Build history of the part. All positions in model axes, mm. A direction names the side the tool comes from. Give positions to 0.01 mm unless a question says otherwise; leave off trailing zeros. Write item = value, one per line. Start each with the question number.
Q1. Mould opens along Y. For faces 1 (the face through (62.12, 0.04, 3.13)), 2 (the face through (-12.17, 78.12, 3.13)), 3 (the face through (-38.56, 46.17, 3.13)), 4 (the face through (1, 3, 6.35)) say: pulls with the +Y half, pulls with the -Y half, needs draft (parallel to the pull), parting line crosses it, or undercut.
Q2. Drop flat-ended pins along their axis: P1, Ø4, axis at x = -28.5, y = -54.2, coming from the -Z side; P2, Ø2, axis at x = -41.5, z = 5.5, coming from the +Y side; P3, Ø3, axis at x = 43.5, z = 4.5, coming from the +Y side. Give the stop position or say it passes through.
Q3. Tool access for faces 5 (the face through (1, 3, 0)), 6 (the face through (-33.757, -32.465, 3.131)): list every direction of +Z, -Z, +X, -X, +Y, -Y with a clear straight run to the whole face (end or side of a thin tool).
Q4. Wall check: line 1 (X direction, y = -31, z = 3.5); line 2 (Y direction, x = -18.5, z = 4.5); line 3 (Y direction, x = 28, z = 5). Give the ranges that are in metal, low to high.
Q5. Saw through at A-A, the plane z = 1.25. Give the number of separate pieces and of enclosed holes in the cut face, then the cut area to 3 significant figures.
from build123d import *

# Parameters (mm, degrees)
MODEL_R             = 1.45
MODEL_R_2           = 1.55
MODEL_R_3           = 3.3
MODEL_R_4           = 3.048
BOSS_EXTRUDE1_DEPTH = 6.35


with BuildPart() as part:
    # Model → Boss-Extrude1 (new body)
    with BuildSketch(Plane.XY):
        with BuildLine():
            ThreePointArc((71.963132539, -16.30426092), (71.896606956, -19.345127891), (73.024752162, -22.169766979))
            ThreePointArc((73.024752162, -22.169766979), (73.705673151, -28.611226497), (68.857053859, -32.906217194))
            ThreePointArc((68.857053859, -32.906217194), (66.118599711, -34.22991144), (64.11603721, -36.519243442))
            ThreePointArc((64.11603721, -36.519243442), (11.268864031, -72.921423961), (-50.101470416, -54.169770455))
            ThreePointArc((-50.101470416, -54.169770455), (-52.70167567, -52.591724124), (-55.71195748, -52.156406987))
            ThreePointArc((-55.71195748, -52.156406987), (-61.630885553, -49.525372103), (-62.92614696, -43.178849276))
            ThreePointArc((-62.92614696, -43.178849276), (-62.703272731, -40.145431292), (-63.684611152, -37.266495293))
            ThreePointArc((-63.684611152, -37.266495293), (-68.786237646, 26.701589457), (-21.861662123, 70.474031375))
            ThreePointArc((-21.861662123, 70.474031375), (-19.194931286, 71.936852015), (-17.312794682, 74.326173966))
            ThreePointArc((-17.312794682, 74.326173966), (-12.074787597, 78.1365986), (-5.930906899, 76.08506647))
            ThreePointArc((-5.930906899, 76.08506647), (-3.41532698, 74.375342732), (-0.431426057, 73.785738734))
            ThreePointArc((-0.431426057, 73.785738734), (57.517373614, 46.219834503), (71.963132539, -16.30426092))
        make_face()
        with Locations((-10.994529329, 71.146189371)):
            Circle(MODEL_R, mode=Mode.SUBTRACT)
        with Locations((-56.117142713, -45.094636387)):
            Circle(MODEL_R, mode=Mode.SUBTRACT)
        with Locations((-4.695418168, 60.932414429)):
            Circle(MODEL_R, mode=Mode.SUBTRACT)
        with Locations((-31.422079216, 58.547967052)):
            Circle(MODEL_R, mode=Mode.SUBTRACT)
        with Locations((-25.122968055, 48.33419211)):
            Circle(MODEL_R, mode=Mode.SUBTRACT)
        with Locations((-50.421309724, -34.532558628)):
            Circle(MODEL_R, mode=Mode.SUBTRACT)
        with Locations((-34.9929872, -56.486302366)):
            Circle(MODEL_R, mode=Mode.SUBTRACT)
        with Locations((-29.29715421, -45.924224608)):
            Circle(MODEL_R, mode=Mode.SUBTRACT)
        with Locations((67.111672043, -26.051552984)):
            Circle(MODEL_R, mode=Mode.SUBTRACT)
        with Locations((-24.235417087, 18.341485339)):
            Circle(MODEL_R_2, mode=Mode.SUBTRACT)
        with Locations((-5.510157235, 29.889859367)):
            Circle(MODEL_R_2, mode=Mode.SUBTRACT)
        with Locations((-26.507192439, 63.935772611)):
            Circle(MODEL_R_2, mode=Mode.SUBTRACT)
        with Locations((-45.232452291, 52.387398583)):
            Circle(MODEL_R_2, mode=Mode.SUBTRACT)
        with Locations((-22.752591866, -65.366152049)):
            Circle(MODEL_R_2, mode=Mode.SUBTRACT)
        with Locations((-42.116407073, -54.923788341)):
            Circle(MODEL_R_2, mode=Mode.SUBTRACT)
        with Locations((-3.766483704, -30.159229537)):
            Circle(MODEL_R_2, mode=Mode.SUBTRACT)
        with Locations((-23.130298911, -19.716865827)):
            Circle(MODEL_R_2, mode=Mode.SUBTRACT)
        with Locations((28.001900788, 11.817744198)):
            Circle(MODEL_R_2, mode=Mode.SUBTRACT)
        with Locations((28.640456145, -10.17299354)):
            Circle(MODEL_R_2, mode=Mode.SUBTRACT)
        with Locations((68.623599511, -9.01198427)):
            Circle(MODEL_R_2, mode=Mode.SUBTRACT)
        with Locations((67.985044157, 12.978753468)):
            Circle(MODEL_R_2, mode=Mode.SUBTRACT)
        with Locations((27.199561986, -44.103080206)):
            Circle(MODEL_R_3, mode=Mode.SUBTRACT)
        with Locations((24.594606851, 45.607051755)):
            Circle(MODEL_R_3, mode=Mode.SUBTRACT)
        with Locations((-51.794168837, -1.503971549)):
            Circle(MODEL_R_3, mode=Mode.SUBTRACT)
        with Locations((-13.480814628, -1.823331492)):
            Circle(MODEL_R_4, mode=Mode.SUBTRACT)
        with Locations((5.883000578, -12.265695202)):
            Circle(MODEL_R_4, mode=Mode.SUBTRACT)
        with Locations((24.86910874, 22.94122731)):
            Circle(MODEL_R_4, mode=Mode.SUBTRACT)
        with Locations((5.505293533, 33.38359102)):
            Circle(MODEL_R_4, mode=Mode.SUBTRACT)
        with Locations((54.420122264, -2.409967499)):
            Circle(MODEL_R, mode=Mode.SUBTRACT)
        with Locations((66.415066415, -2.061664685)):
            Circle(MODEL_R, mode=Mode.SUBTRACT)
        with Locations((55.116727894, -26.399855798)):
            Circle(MODEL_R, mode=Mode.SUBTRACT)
        with BuildLine():
            Line((-34.947891278, 52.97654312), (-42.273098177, 39.165528758))
            Line((-42.273098177, 39.165528758), (-38.099417944, 36.951855639))
            Line((-38.099417944, 36.951855639), (-31.90308597, 48.634478542))
            ThreePointArc((-31.90308597, 48.634478542), (-31.465095291, 49.320977327), (-30.923040746, 49.928672388))
            ThreePointArc((-30.923040746, 49.928672388), (-31.145027643, 53.816962234), (-34.947891278, 52.97654312))
        make_face(mode=Mode.SUBTRACT)
        with BuildLine():
            Line((63.352977787, 3.777490095), (55.054891945, 17.02681254))
            Line((55.054891945, 17.02681254), (51.050954672, 14.519135991))
            Line((51.050954672, 14.519135991), (58.070236902, 3.311643638))
            ThreePointArc((58.070236902, 3.311643638), (58.44576695, 2.589083191), (58.701019038, 1.815802654))
            ThreePointArc((58.701019038, 1.815802654), (62.179370269, 0.06390403), (63.352977787, 3.777490095))
        make_face(mode=Mode.SUBTRACT)
        with BuildLine():
            Line((-28.40508651, -56.754033215), (-12.781793768, -56.192341298))
            Line((-12.781793768, -56.192341298), (-12.951536728, -51.47099163))
            Line((-12.951536728, -51.47099163), (-26.167150935, -51.946122181))
            ThreePointArc((-26.167150935, -51.946122181), (-26.980671662, -51.910060518), (-27.777978294, -51.744475042))
            ThreePointArc((-27.777978294, -51.744475042), (-31.034342627, -53.880866258), (-28.40508651, -56.754033215))
        make_face(mode=Mode.SUBTRACT)
        Polygon((53.043356097, -5.945390314), (44.795552885, -6.184885641), (45.197066243, -20.012308543), (53.444869455, -19.772813215), align=None, mode=Mode.SUBTRACT)
        Polygon((-21.372819002, 48.909589039), (-17.041508358, 41.886529595), (-5.267365536, 49.147961813), (-9.598676177, 56.171021257), align=None, mode=Mode.SUBTRACT)
        Polygon((-31.670537096, -42.964198725), (-27.754044527, -35.701643953), (-39.929700707, -29.13565327), (-43.846193278, -36.398208042), align=None, mode=Mode.SUBTRACT)
    extrude(amount=BOSS_EXTRUDE1_DEPTH)


solid = part.part
Report:
q1.face_1 = undercut
q1.face_2 = pulls with the +Y half
q1.face_3 = undercut
q1.face_4 = needs draft
q2.P1 = through
q2.P2 = 61.68
q2.P3 = 60.67
q3.face_5 = -Z, +X, -X, +Y, -Y
q3.face_6 = +Z, -Z
q4.line_1 = -66.96 to -40.94, -36.47 to -5.07, -2.46 to 72.17
q4.line_2 = -71.43 to -56.4, -51.67 to 44.25, 50.68 to 72.61
q4.line_3 = -68.27 to -47.3, -40.9 to -11.58, -8.76 to 10.27, 13.37 to 68.27
q5.separate_pieces = 1
q5.enclosed_holes = 37
q5.area = 16,300 mm2
